Autodesk Inventor part; units mm, degrees
ref_plane "YZ Plane" through (0, 0, 0) normal (1, 0, 0) x (0, 1, 0)
ref_plane "XZ Plane" through (0, 0, 0) normal (0, 1, 0) x (-1, 0, 0)
ref_plane "XY Plane" through (0, 0, 0) normal (0, 0, 1) x (1, 0, 0)
ref_plane "Work Plane1" through (0, 0, 0) normal (0, 0, 1) x (1, 0, 0)
sketch "Sketch1" plane through (0, 0, 0) normal (0, 0, 1) x (1, 0, 0)
  circle A0 centre (3, -74.8889) radius 2.3
  line L0 (3, 0) -> (3, -44.7889)
  line L1 (0, 0) -> (3, 0)
  line L2 (0, -77.8889) -> (0, 0)
  line L3 (0, -77.8889) -> (6, -77.8889)
  line L4 (6, -71.8889) -> (6, -77.8889)
  line L5 (6, -71.8889) -> (1.6, -71.8889)
  line L6 (1.6, -71.8889) -> (1.6, -56.7889)
  line L7 (1.6, -56.7889) -> (9.6, -56.7889)
  line L8 (9.6, -44.7889) -> (9.6, -56.7889)
  line L9 (3, -44.7889) -> (9.6, -44.7889)
  circle A1 centre (5.6, -52.7889) radius 2.6
  circle A2 centre (172.4, -49.8889) radius 2.6
  circle A3 centre (175, -74.8889) radius 2.3
  line L10 (168.4, -41.8889) -> (175, -41.8889)
  line L11 (168.4, -53.8889) -> (168.4, -41.8889)
  line L12 (175, -53.8889) -> (168.4, -53.8889)
  line L13 (175, -53.8889) -> (175, -71.8889)
  line L14 (175, -71.8889) -> (172, -71.8889)
  line L15 (172, -71.8889) -> (172, -77.8889)
  line L16 (178, -77.8889) -> (172, -77.8889)
  line L17 (178, -77.8889) -> (178, 0)
  line L18 (178, 0) -> (175, 0)
  line L19 (175, 0) -> (175, -41.8889)
  line L20 (65.5, 41.9823) -> (65.5, 55)
  line L21 (112.5, 41.9823) -> (112.5, 55)
  line L22 (62.4925, 0) -> (3, 0)
  line L23 (115.5075, 0) -> (175, 0)
  line L24 (65.5, 55) -> (112.5, 55)
  line L25 (112.5, 55) -> (112.5, 0)
  line L26 (112.5, 0) -> (65.5, 0)
  line L27 (65.5, 0) -> (65.5, 55)
  line L28 (178, 0) -> (0, 0)
  line L29 (0, 0) -> (0, -77.8889)
  line L30 (0, -77.8889) -> (178, -77.8889)
  line L31 (178, -77.8889) -> (178, 0)
  line L32 (31.25, -62.8889) -> (31.25, -73.8889)
  line L33 (31.25, -73.8889) -> (57.25, -73.8889)
  line L34 (57.25, -73.8889) -> (57.25, -62.8889)
  line L35 (57.25, -62.8889) -> (31.25, -62.8889)
  line L36 (21.2501, -70.339) -> (21.2501, -58.3388)
  line L37 (21.2501, -58.3388) -> (3.2499, -58.3388)
  line L38 (3.2499, -70.339) -> (21.2501, -70.339)
  line L39 (3.2499, -58.3388) -> (3.2499, -70.339)
  line L40 (156.2, -70.4889) -> (156.2, -59.9889)
  line L41 (166.7, -59.9889) -> (156.2, -59.9889)
  line L42 (166.7, -59.9889) -> (166.7, -70.4889)
  line L43 (156.2, -70.4889) -> (166.7, -70.4889)
  line L44 (149, -59.8889) -> (149, -70.8889)
  line L45 (149, -70.8889) -> (136.35, -70.8889)
  line L46 (136.35, -70.8889) -> (136.35, -59.8889)
  line L47 (136.35, -59.8889) -> (149, -59.8889)
  line L48 (135, -53.8889) -> (135, -71.8889)
  line L49 (135, -71.8889) -> (175, -71.8889)
  line L50 (175, -71.8889) -> (175, -53.8889)
  line L51 (175, -53.8889) -> (135, -53.8889)
  circle A4 centre (137.85, -56.7389) radius 1.5
  circle A5 centre (172.15, -56.7389) radius 1.5
  line L52 (2.2499, -57.3388) -> (22.2501, -57.3388)
  line L53 (22.2501, -57.3388) -> (22.2501, -71.339)
  line L54 (22.2501, -71.339) -> (2.2499, -71.339)
  line L55 (2.2499, -71.339) -> (2.2499, -57.3388)
  line L56 (30.25, -61.8889) -> (30.25, -74.8889)
  line L57 (30.25, -74.8889) -> (58.25, -74.8889)
  line L58 (58.25, -74.8889) -> (58.25, -61.8889)
  line L59 (58.25, -61.8889) -> (30.25, -61.8889)
  line L60 (155.2, -58.9889) -> (155.2, -71.4889)
  line L61 (155.2, -71.4889) -> (167.7, -71.4889)
  line L62 (167.7, -71.4889) -> (167.7, -58.9889)
  line L63 (167.7, -58.9889) -> (155.2, -58.9889)
  line L64 (150, -58.8889) -> (150, -71.8889)
  line L65 (150, -71.8889) -> (135.35, -71.8889)
  line L66 (135.35, -71.8889) -> (135.35, -58.8889)
  line L67 (135.35, -58.8889) -> (150, -58.8889)
  dimension "d0" = 1
  dimension "d1" = 1
  dimension "d2" = 1
  dimension "d3" = 1
extrude "Extrusion1" add sketch "Sketch1" along normal blind 2 contours A0 | L22 L28 L26 L23 L19 L10 L11 L51 L48 L49 L15 L30 L4 L5 L6 L7 L8 L9 L0 | L0 L9 L8 L7 L6 L5 L4 L3 L2 L1 | L27 L20 L24 L21 L25 L26 | L15 L14 L13 L12 L11 L10 L19 L18 L17 L16 | L49 L64 L67 L66 L48 L51 L12 L13 L14 | A1 | A2 | A3 | A4 | A5
sketch "Sketch2" plane through (0, 0, 2) normal (0, 0, 1) x (1, 0, 0)
  circle A0 centre (3, -74.8889) radius 2
  circle A1 centre (5.6, -52.7889) radius 2.6
  circle A2 centre (172.4, -49.8889) radius 2.6
  circle A3 centre (175, -74.8889) radius 2
  circle A4 centre (108.4457, 27.5) radius 2.3
  circle A5 centre (69.5, 27.5) radius 2.3
  circle A6 centre (69.5, 4.0875) radius 2.3
  circle A7 centre (108.4841, 4.0875) radius 2.3
  circle A8 centre (89, -0.5003) radius 2.3
  circle A9 centre (89, 27.5) radius 2.3
  point P0 (0, 0)
hole "Hole1" at (3, -74.8889, 2) at (5.6, -52.7889, 2) at (175, -74.8889, 2) at (172.4, -49.8889, 2) at (89, -0.5003, 2) at (69.5, 4.0875, 2) at (108.4841, 4.0875, 2) at (89, 27.5, 2) at (69.5, 27.5, 2) at (108.4457, 27.5, 2) direction (0, 0, -1) diameter 3.6 end through all countersink diameter 6.3 countersink angle 90
properties part number "ceil"
Could you check a few things on this model? Use its own coordinates, in mm. Coordinates: 2 decimals unless noted, no trailing zeros. Order: outer loops, then holes, each group sorted by start corner. A loop starts at its lowest first (then second) coordinate and runs counter-clockwise, first axis right, second up. Notation, with made-up numbers: M 9.25,43.25 L 31.25,43.25 A17 ccw 31.25,71.25 Z; hole C 81,-37 d3. An arc over 180 degrees is marked long. Use a Markdown table: item, result. Add a question column.
Q1. I want a section at C-C on x = 124. List the corners of the cut face in (y, z) for me, then the cut area to 3 significant figures.
Q2. I'm going to push flat-ended pins straight in: pin 1 (3 mm diameter, centred on x = 175, y = -74.89, fed in from +Z); pin 2 (1 mm diameter, centred on x = 27.5, z = 1, fed in from +Y). Where does each tip first touch, or does it pass through?
Q3. I want a section at A-A on y = 27.5. List the corners of the cut face in (x, z) for me, then the cut area to 3 significant figures.
Q4. I want a section at B-B on x = 89. List the corners of the cut face in (y, z) for me.
Q5. We'd pull the mould along X, two halves only. Please class faces 1 (the flat face through (88, -25, 2)), 2 (the conical face through (109, 2, 1)): pulls with the +X half, pulls with the -X half, needs draft (parallel to the pull), parting line crosses it, or undercut.
Q6. If I drill on L1, parallel to X at y = -59.5, z = 1.45; L2, parallel to Y at x = 89, z = 0.45; L3, parallel to Y at x = 31.5, z = 1.6, over which ranges is the centre line in solid material (lowest first)?
Checked values:
| question | item | result |
|---|---|---|
| 1 | outline | M -77.89,0 L 0,0 L 0,2 L -77.89,2 Z |
| 1 | area | 156 mm² |
| 2 | pin 1 | through |
| 2 | pin 2 | y = 0 |
| 3 | outline | M 65.5,0 L 67.7,0 L 67.7,0.65 L 66.35,2 L 65.5,2 Z; M 71.3,0 L 87.2,0 L 87.2,0.65 L 85.85,2 L 72.65,2 L 71.3,0.65 Z; M 90.8,0 L 106.65,0 L 106.65,0.65 L 105.3,2 L 92.15,2 L 90.8,0.65 Z; M 110.25,0 L 112.5,0 L 112.5,2 L 111.6,2 L 110.25,0.65 Z |
| 3 | area | 66.9 mm² |
| 4 | outline | M -77.89,0 L -2.3,0 L -2.3,0.65 L -3.65,2 L -77.89,2 Z; M 1.3,0 L 25.7,0 L 25.7,0.65 L 24.35,2 L 2.65,2 L 1.3,0.65 Z; M 29.3,0 L 55,0 L 55,2 L 30.65,2 L 29.3,0.65 Z |
| 5 | face 1 | needs draft |
| 5 | face 2 | undercut |
| 6 | L1 | 0 to 2.25, 22.25 to 135.35, 150 to 155.2, 167.7 to 178 |
| 6 | L2 | -77.89 to -2.3, 1.3 to 25.7, 29.3 to 55 |
| 6 | L3 | -77.89 to -74.89, -61.89 to 0 |
